The listing builds one solid part. Answer for the finished solid, in the listing's coordinates (mm). Face numbers are marked on the shaded views. A direction names the side the tool comes from. Coordinates: 2 decimals unless noted, no trailing zeros. Order: outer loops, then holes, each group sorted by start corner. A loop starts at its lowest first (then second) coordinate and runs counter-clockwise, first axis right, second up. Notation, with made-up numbers: (-34, 3) -> (2, 3) arc R27 cw to (2, 37) -> close; hole circle Ø11 at (5.25, -29). An arc over 180 degrees is marked (long way). Write item = value, one per line. Start each with the question number.
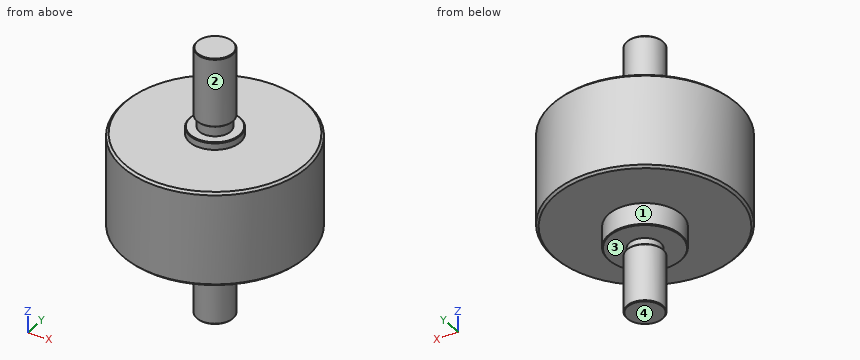
Autodesk Inventor part; units mm, degrees
ref_plane "YZ Plane" through (0, 0, 0) normal (1, 0, 0) x (0, 1, 0)
ref_plane "XZ Plane" through (0, 0, 0) normal (0, 1, 0) x (-1, 0, 0)
ref_plane "XY Plane" through (0, 0, 0) normal (0, 0, 1) x (1, 0, 0)
sketch "Sketch1" plane through (0, 0, 0) normal (0, 0, 1) x (1, 0, 0)
  circle A0 centre (0, 0) radius 12.7
  dimension "d0" = 25.4
extrude "Extrusion1" add sketch "Sketch1" along normal blind 13
sketch "Sketch2" plane through (0, 0, 13) normal (0, 0, 1) x (1, 0, 0)
  circle A0 centre (0, 0) radius 2.5
  dimension "d3" = 5
extrude "Extrusion2" add sketch "Sketch2" along normal blind 12
sketch "Sketch3" plane through (0, 0, 0) normal (0, 0, -1) x (-1, 0, 0)
  circle A0 centre (0, 0) radius 2.5
  dimension "d6" = 5
extrude "Extrusion3" add sketch "Sketch3" along normal blind 12
sketch "Sketch4" plane through (0, 0, 13) normal (0, 0, 1) x (1, 0, 0)
  circle A0 centre (0, 0) radius 2.15
  circle A1 centre (0, 0) radius 3.5
  dimension "d9" = 4.3
  dimension "d10" = 7
extrude "Extrusion4" cut sketch "Sketch4" along normal blind 2.5
sketch "Sketch5" plane through (0, 0, 0) normal (0, 0, -1) x (-1, 0, 0)
  circle A0 centre (0, 0) radius 3
  circle A1 centre (0, 0) radius 2.15
  dimension "d13" = 6
  dimension "d14" = 4.3
extrude "Extrusion5" cut sketch "Sketch5" along normal blind 4
sketch "Sketch6" plane through (0, 0, 13) normal (0, 0, 1) x (1, 0, 0)
  circle A0 centre (0, 0) radius 3.5
  dimension "d17" = 7
extrude "Extrusion6" add sketch "Sketch6" along normal blind 1
sketch "Sketch7" plane through (0, 0, 0) normal (0, 0, -1) x (-1, 0, 0)
  circle A0 centre (0, 0) radius 5
  dimension "d20" = 10
extrude "Extrusion7" add sketch "Sketch7" along normal blind 3
chamfer "Chamfer1" distance 0.1 angle 45 6 edges at (-2.5, 0, 25) (-2.5, 0, 15.5) (-3.5, 0, 14) (2.5, 0, -12) (2.5, 0, -4) (5, 0, -3)
chamfer "Chamfer2" distance 0.3 angle 45 2 edges at (-12.7, 0, 13) (-12.7, 0, 0)
thread "Thread1"
thread "Thread2"
properties part number "Force_Sensor"
Item 1: Each of these flat-tipped pins is pushed along its axis until it touches: pin 1 (3 mm diameter, centred on y = 1.5, z = 7.5, fed in from +X); pin 2 (6 mm diameter, centred on y = -5, z = 3.5, fed in from +X); pin 3 (2 mm diameter, centred on y = 10, z = 9, fed in from +X); pin 4 (12 mm diameter, centred on x = -6.5, z = 12, fed in from +Y). Where does it stop, or does it pass through?
Item 2: Section A-A, the plane z = 7.5 is taken. Give the vertices of the cut face in (x, y), then the cut area to 3 significant figures.
Item 3: Consider probe 1 along Z at (x, y) = (4.5, 9.5); probe 2 along X at (y, z) = (-2.75, 0.5); probe 3 along Z at (x, y) = (3, -0.75). Determine where each line is inside the solid, lowest interval first.
Item 4: Which of the six approach directions +Z, -Z, +X, -X, +Y, -Y give full straight-line access (tool end or side, diameter ignored) to the marked faces 1, 2, 3 and 4?
A:
q1.pin_1 = 12.7
q1.pin_2 = 12.54
q1.pin_3 = 8.96
q1.pin_4 = 12.69
q2.outline = circle Ø25.4 at (0, 0)
q2.area = 507 mm^2
q3.probe_1 = 0 to 13
q3.probe_2 = -12.4 to 12.4
q3.probe_3 = -3 to 14
q4.face_1 = -Z
q4.face_2 = +Z
q4.face_3 = none
q4.face_4 = -Z, +X, -X, +Y, -Y
